Geometry check sheet. Reference: drawing and pictorial views, mm from the part's lowest x, y, z. A direction names the side the tool comes from. Round coordinates to 2 decimals unless told otherwise and drop trailing zeros. Loops run counter-clockwise (first coordinate to the right, second up) from the corner with the lowest first, then second, coordinate; pieces in that order, holes last. Notation, with made-up numbers: (43, 38) - (71, 38) arc R22 cw to (71, 49) - close; hole circle Ø1 at (-39, -33.5). An arc over 180 degrees is marked (long way). Return JSON: item names as keys, results as strings.
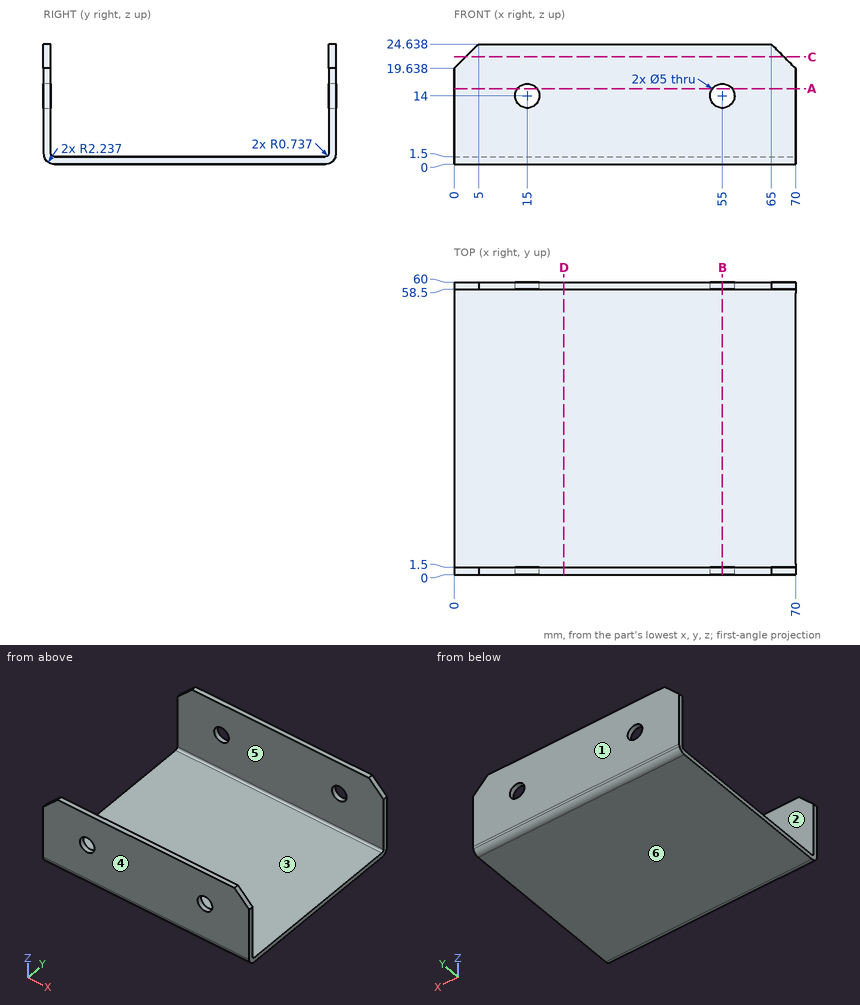
Q1. Sectioned sample at B-B (x = 55). Enter the section's corners in (y, z) (1 decimal).
Answer key:
{"outline": "(0, 2.2) arc R2.2 ccw to (2.2, 0) - (57.8, 0) arc R2.2 ccw to (60, 2.2) - (60, 11.5) - (58.5, 11.5) - (58.5, 2.2) arc R0.7 cw to (57.8, 1.5) - (2.2, 1.5) arc R0.7 cw to (1.5, 2.2) - (1.5, 11.5) - (0, 11.5) - close; (0, 16.5) - (1.5, 16.5) - (1.5, 24.6) - (0, 24.6) - close; (58.5, 16.5) - (60, 16.5) - (60, 24.6) - (58.5, 24.6) - close"}
Q2. Tool access check on the marked faces 1 and 2. Record the directions out of +Z, -Z, +X, -X, +Y, -Y that give a thin tool (end or side, any length) a straight path to the whole face; none if there is none.
Answer key:
{"face 1": "+Z, -Z, +X, -X, +Y", "face 2": "+Z, +X, -X"}
Q3. Sectioned sample at A-A (z = 15.5). Enter the section's corners in (x, y).
Answer key:
{"outline": "(0, 0) - (13, 0) - (13, 1.5) - (0, 1.5) - close; (0, 58.5) - (13, 58.5) - (13, 60) - (0, 60) - close; (17, 0) - (53, 0) - (53, 1.5) - (17, 1.5) - close; (17, 58.5) - (53, 58.5) - (53, 60) - (17, 60) - close; (57, 0) - (70, 0) - (70, 1.5) - (57, 1.5) - close; (57, 58.5) - (70, 58.5) - (70, 60) - (57, 60) - close"}
Q4. Sectioned sample at D-D (x = 22.5). Enter the section's corners in (y, z) (1 decimal).
Answer key:
{"outline": "(0, 2.2) arc R2.2 ccw to (2.2, 0) - (57.8, 0) arc R2.2 ccw to (60, 2.2) - (60, 24.6) - (58.5, 24.6) - (58.5, 2.2) arc R0.7 cw to (57.8, 1.5) - (2.2, 1.5) arc R0.7 cw to (1.5, 2.2) - (1.5, 24.6) - (0, 24.6) - close"}
Q5. Sectioned sample at C-C (z = 22). Enter the section's corners in (x, y).
Answer key:
{"outline": "(2.36, 0) - (67.64, 0) - (67.64, 1.5) - (2.36, 1.5) - close; (2.36, 58.5) - (67.64, 58.5) - (67.64, 60) - (2.36, 60) - close"}
Q6. Scan lines: probe 1 along X at (y, z) = (59.3, 14); probe 2 along Y at (x, z) = (29.5, 9.75); probe 3 along Z at (x, y) = (31.5, 28.5). Record each from-to range of solid material in increasing order. Write a range as [from, to].
Answer key:
{"probe 1": "x = [0, 12.5], [17.5, 52.5], [57.5, 70]", "probe 2": "y = [0, 1.5], [58.5, 60]", "probe 3": "z = [0, 1.5]"}
Q7. Draft check along Y on the marked faces 3, 4, 5 and 6. Enter one of: released by +Y, released by -Y, zero draft, split by the parting line, or undercut.
Answer key:
{"face 3": "undercut", "face 4": "released by -Y", "face 5": "undercut", "face 6": "zero draft"}
Q8. Depth check by flat-ended pin: P1, Ø3, axis at x = 15, z = 14, coming from the +Y side. Enter the tip coordinate at first touch or a pass-through.
Answer key:
{"P1": "passes through"}
